Model file for the job. Use its own axes, mm. Face numbers are marked on the shaded views. A direction names the side the tool comes from. Give positions to 0.01 mm unless a question says otherwise; leave off trailing zeros. Order: outer loops, then holes, each group sorted by start corner. A loop starts at its lowest first (then second) coordinate and runs counter-clockwise, first axis right, second up. Notation, with made-up numbers: (24, 79) -> (60, 79) arc R4 cw to (60, 85) -> close; hole circle Ø4 at (-23.75, 31). An arc over 180 degrees is marked (long way). Use CSV: the item, a comma, the result in double quotes. Start each with the question number.
1. 3-axis set-ups, long thin cutter, end or side, ignore diameter. For the marked faces 4 and 5: which of +Z, -Z, +X, -X, +Y, -Y reach the whole face in a straight line?
2. Wall check: line 1 (X direction, y = 63, z = 0); line 2 (X direction, y = 63.5, z = 13.5); line 3 (Y direction, x = 13.5, z = -6.5). Give the ranges that are in metal, low to high. Write a range as from..to.
3. Cut at B-B on x = 0. List the corners of the cut face in (y, z), then the cut area to 3 significant figures.
4. Cut at D-D on x = 4.5. List the corners of the cut face in (y, z).
5. Drop flat-ended pins along their axis: pin 1 (2.5 mm diameter, centred on x = 0.5, y = 82, fed in from -Z); pin 2 (8 mm diameter, centred on y = 23.5, z = -12, fed in from -X); pin 3 (4 mm diameter, centred on y = 10, z = -5.5, fed in from -X). Give the stop position or say it passes through.
6. Pull direction Y, two halves, no side cores. Call the marked faces 1, 2 and 3: released by +Y, released by -Y, zero draft, split by the parting line, or undercut.
7. Cut at C-C on y = 24. List the corners of the cut face in (x, z).
8. Cut at A-A on z = 0. List the corners of the cut face in (x, y), then the cut area to 3 significant figures.
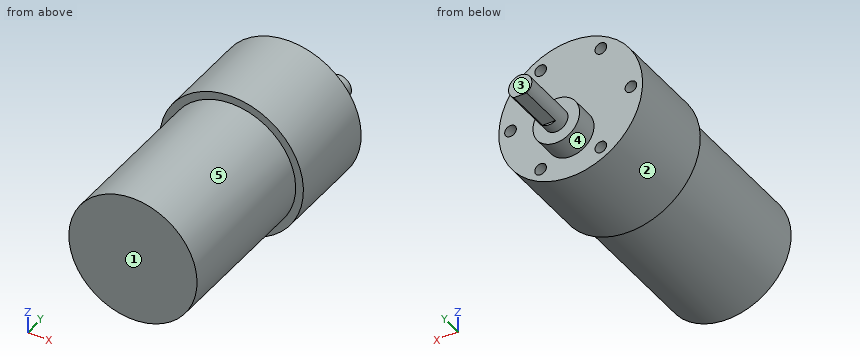
```python
from build123d import *

# Parameters (mm, degrees)
SKETCH1_R           = 16.5
BOSS_EXTRUDE1_DEPTH = 41
SKETCH2_R           = 18.5
BOSS_EXTRUDE2_DEPTH = 24
SKETCH3_R           = 6
BOSS_EXTRUDE3_DEPTH = 6
SKETCH4_R           = 3
BOSS_EXTRUDE4_DEPTH = 15
SKETCH5_W           = 8.086329314
SKETCH5_H           = 5.281822038
CUT_EXTRUDE1_DEPTH  = 12
SKETCH6_R           = 1.5
CUT_EXTRUDE2_DEPTH  = 3


with BuildPart() as part:
    # Sketch1 → Boss-Extrude1 (new body)
    with BuildSketch(Plane(origin=(0, 0, 0), x_dir=(1, 0, 0), z_dir=(0, 1, 0))):
        with Locations(Location((0, 0, 0), (0, 0, 270))):
            Circle(SKETCH1_R)
    extrude(amount=BOSS_EXTRUDE1_DEPTH)

    # Sketch2 → Boss-Extrude2 (add)
    with BuildSketch(Plane(origin=(0, 41, 0), x_dir=(1, 0, 0), z_dir=(0, 1, 0))):
        with Locations(Location((0, 0, 0), (0, 0, 270))):
            Circle(SKETCH2_R)
    extrude(amount=BOSS_EXTRUDE2_DEPTH)

    # Sketch3 → Boss-Extrude3 (add)
    with BuildSketch(Plane(origin=(0, 65, 0), x_dir=(1, 0, 0), z_dir=(0, 1, 0))):
        with Locations(Location((0, 7, 0), (0, 0, 270))):
            Circle(SKETCH3_R)
    extrude(amount=BOSS_EXTRUDE3_DEPTH)

    # Sketch4 → Boss-Extrude4 (add)
    with BuildSketch(Plane(origin=(0, 71, 0), x_dir=(1, 0, 0), z_dir=(0, 1, 0))):
        with Locations(Location((0, 7, 0), (0, 0, 270))):
            Circle(SKETCH4_R)
    extrude(amount=BOSS_EXTRUDE4_DEPTH)

    # Sketch5 → Cut-Extrude1 (cut)
    with BuildSketch(Plane(origin=(0, 86, 0), x_dir=(1, 0, 0), z_dir=(0, 1, 0))):
        with Locations((0.101264993, 12.140911019)):
            Rectangle(SKETCH5_W, SKETCH5_H)
    extrude(amount=-CUT_EXTRUDE1_DEPTH, mode=Mode.SUBTRACT)

    # Sketch6 → Cut-Extrude2 (cut)
    with BuildSketch(Plane(origin=(0, 65, 0), x_dir=(1, 0, 0), z_dir=(0, 1, 0))):
        with Locations(Location((-15.5, 0, 0), (0, 0, 270))):
            Circle(SKETCH6_R)
        with Locations(Location((-7.75, 13.423393759, 0), (0, 0, 270))):
            Circle(SKETCH6_R)
        with Locations(Location((7.75, 13.423393759, 0), (0, 0, 270))):
            Circle(SKETCH6_R)
        with Locations(Location((15.5, 0, 0), (0, 0, 270))):
            Circle(SKETCH6_R)
        with Locations(Location((7.75, -13.423393759, 0), (0, 0, 270))):
            Circle(SKETCH6_R)
        with Locations(Location((-7.75, -13.423393759, 0), (0, 0, 270))):
            Circle(SKETCH6_R)
    extrude(amount=-CUT_EXTRUDE2_DEPTH, mode=Mode.SUBTRACT)


solid = part.part
```
Verdict:
1,face 4,"+Y"
1,face 5,"-Y"
2,line 1,"-18.5..-17, -14..14, 17..18.5"
2,line 2,"-12.65..-9.25, -6.25..6.25, 9.25..12.65"
2,line 3,"0..65"
3,outline,"(0, -16.5) -> (41, -16.5) -> (41, -18.5) -> (65, -18.5) -> (65, -13) -> (71, -13) -> (71, -10) -> (74, -10) -> (74, -9.5) -> (86, -9.5) -> (86, -4) -> (71, -4) -> (71, -1) -> (65, -1) -> (65, 18.5) -> (41, 18.5) -> (41, 16.5) -> (0, 16.5) -> close"
3,area,"2,400 mm^2"
4,outline,"(0, -15.87) -> (41, -15.87) -> (41, -17.94) -> (65, -17.94) -> (65, -10.97) -> (71, -10.97) -> (71, -3.03) -> (65, -3.03) -> (65, 17.94) -> (41, 17.94) -> (41, 15.87) -> (0, 15.87) -> close"
5,pin 1,"z = -9.5"
5,pin 2,"x = -14.43"
5,pin 3,"x = -16.12"
6,face 1,"released by -Y"
6,face 2,"zero draft"
6,face 3,"released by +Y"
7,outline,"circle Ø33 at (0, 0)"
8,outline,"(-18.5, 41) -> (-16.5, 41) -> (-16.5, 0) -> (16.5, 0) -> (16.5, 41) -> (18.5, 41) -> (18.5, 65) -> (17, 65) -> (17, 62) -> (14, 62) -> (14, 65) -> (-14, 65) -> (-14, 62) -> (-17, 62) -> (-17, 65) -> (-18.5, 65) -> close"
8,area,"2,220 mm^2"
